from build123d import *

# Parameters (mm, degrees)
F1_DEPTH = 3.175


# Not quite as in the source:
# - a feature names something its author has since deleted; it is built from what else it names


with BuildPart() as f1:
    # F0 (on Front) → F1 (new body)
    with BuildSketch(Plane.XZ):
        with BuildLine():
            ThreePointArc((0, 3.05), (2.1566756826, 2.1566756826), (3.05, 0))
            ThreePointArc((3.05, 0), (2.1566756826, -2.1566756826), (0, -3.05))
            Line((0, -3.05), (0, -4.9800602682))
            ThreePointArc((0, -4.9800602682), (5.7417944409, -6.7685559702), (9.4194688927, -11.5268782485))
            ThreePointArc((9.4194688927, -11.5268782485), (10.31824899, -10.0042357535), (10.6308735731, -8.2639737901))
            Line((10.6308735731, -8.2639737901), (10.6308735731, 8.2639737901))
            ThreePointArc((10.6308735731, 8.2639737901), (10.3103808484, 10.0252834336), (9.389988909, 11.5607983065))
            ThreePointArc((9.389988909, 11.5607983065), (5.7274768906, 6.8026828494), (0, 5))
            Line((0, 5), (0, 3.05))
        make_face()
        with BuildLine():
            ThreePointArc((0, -3.05), (-3.05, 0), (0, 3.05))
            Line((0, 3.05), (0, 5))
            ThreePointArc((0, 5), (-5.7423447428, 6.8130911295), (-9.4024106226, 11.5949046291))
            ThreePointArc((-9.4024106226, 11.5949046291), (-10.3983579477, 10.0170839844), (-10.7465008538, 8.183992176))
            Line((-10.7465008538, 8.183992176), (-10.7465008538, -8.183992176))
            ThreePointArc((-10.7465008538, -8.183992176), (-10.3930329558, -10.0305401514), (-9.3826050837, -11.6160099542))
            ThreePointArc((-9.3826050837, -11.6160099542), (-5.739751248, -6.8156278258), (0, -4.9800602682))
            Line((0, -4.9800602682), (0, -3.05))
        make_face()
        with BuildLine():
            ThreePointArc((-9.4024106226, 11.5949046291), (-5.7423447428, 6.8130911295), (0, 5))
            Line((0, 5), (0, 15))
            ThreePointArc((0, 15), (-4.5199654888, 14.3027938523), (-8.6197512808, 12.275988264))
            ThreePointArc((-8.6197512808, 12.275988264), (-9.0287945556, 11.9558018286), (-9.4024106226, 11.5949046291))
        make_face()
        with BuildLine():
            Line((0, 15), (0, 5))
            ThreePointArc((0, 5), (5.7274768906, 6.8026828494), (9.389988909, 11.5607983065))
            ThreePointArc((9.389988909, 11.5607983065), (8.9445660683, 12.0082283284), (8.4463103597, 12.3959606852))
            ThreePointArc((8.4463103597, 12.3959606852), (4.4193093195, 14.3342144933), (0, 15))
        make_face()
        with BuildLine():
            ThreePointArc((9.4194688927, -11.5268782485), (5.7417944409, -6.7685559702), (0, -4.9800602682))
            Line((0, -4.9800602682), (0, -15))
            ThreePointArc((0, -15), (4.4193093195, -14.3342144933), (8.4463103597, -12.3959606852))
            ThreePointArc((8.4463103597, -12.3959606852), (8.9613594363, -11.9932986506), (9.4194688927, -11.5268782485))
        make_face()
        with BuildLine():
            Line((0, -15), (0, -4.9800602682))
            ThreePointArc((0, -4.9800602682), (-5.739751248, -6.8156278258), (-9.3826050837, -11.6160099542))
            ThreePointArc((-9.3826050837, -11.6160099542), (-9.0178640795, -11.9652859553), (-8.6197512808, -12.275988264))
            ThreePointArc((-8.6197512808, -12.275988264), (-4.5199654888, -14.3027938523), (0, -15))
        make_face()
        with BuildLine():
            ThreePointArc((-8.6197512808, 12.275988264), (-4.5199654888, 14.3027938523), (0, 15))
            ThreePointArc((0, 15), (4.4193093195, 14.3342144933), (8.4463103597, 12.3959606852))
            ThreePointArc((8.4463103597, 12.3959606852), (8.9445660683, 12.0082283284), (9.389988909, 11.5607983065))
            ThreePointArc((9.389988909, 11.5607983065), (9.8463162932, 13.2535592037), (10, 15))
            ThreePointArc((10, 15), (-1.7285678717, 24.8494696869), (-9.4024106226, 11.5949046291))
            ThreePointArc((-9.4024106226, 11.5949046291), (-9.0287945556, 11.9558018286), (-8.6197512808, 12.275988264))
        make_face()
        with BuildLine():
            ThreePointArc((8.4463103597, -12.3959606852), (4.4193093195, -14.3342144933), (0, -15))
            ThreePointArc((0, -15), (-4.5199654888, -14.3027938523), (-8.6197512808, -12.275988264))
            ThreePointArc((-8.6197512808, -12.275988264), (-9.0178640795, -11.9652859553), (-9.3826050837, -11.6160099542))
            ThreePointArc((-9.3826050837, -11.6160099542), (-1.6724608086, -24.8332220833), (10.0345902517, -14.9800004438))
            ThreePointArc((10.0345902517, -14.9800004438), (9.8796089518, -13.2262596432), (9.4194688927, -11.5268782485))
            ThreePointArc((9.4194688927, -11.5268782485), (8.9613594363, -11.9932986506), (8.4463103597, -12.3959606852))
        make_face()
    extrude(amount=F1_DEPTH)


solid = f1.part
Model file for the job. Use its own axes, mm. A direction names the side the tool comes from. Give positions to 0.01 mm unless a question says otherwise; leave off trailing zeros. Loops run counter-clockwise (first coordinate to the right, second up) from the corner with the lowest first, then second, coordinate; pieces in that order, holes last. Notation, with made-up numbers: (59.5, 72) -> (90.5, 72) arc R17 cw to (90.5, 83) -> close; hole circle Ø7 at (22.5, 66). An arc over 180 degrees is marked (long way). Use a Markdown table: item, result. Add a question column.
(1) Slice it at B-B on z = -16.5. List the corners of the cut face in (x, y) (3 decimals), and give its area (3 significant figures).
(2) Slice it at A-A on y = -2. List the corners of the cut face in (x, z).
(3) Slice it at C-C on x = -3.5. List the corners of the cut face in (y, z) (1 decimal).
(4) Tool access for faces 3 (the flat face through (10.631, -2, 0)), 4 (the cylindrical face through (10.31, -1.57, -10.03)), 5 (the cylindrical face through (-10.39, -1.57, 10.04)): list every direction of +Z, -Z, +X, -X, +Y, -Y with a clear straight run to the whole face (end or side of a thin tool).
(5) Mould opens along Z. For faces 1 (the cylindrical face through (-10.4, -1.57, -10.01)), 2 (the flat face through (5, -3.175, 0)) say: +Z half, -Z half, draft (parallel to the pull), parting line (faces both ways), or undercut.
(6) Wall check: line 1 along X through (y, z) = (-0.7, 1); line 2 along Z through (x, y) = (0.5, -0.2); line 3 along Z through (x, y) = (-0.75, -1.05). Give the ranges that are in metal, low to high.
(7) Drop a flat-ended pin along its axis: pin 1 Ø1 at (x, y) = (1.5, -2) entering from +Z. Give the stop position or say it passes through.
Filled sheet:
| question | item | result |
|---|---|---|
| 1 | outline | (-9.849, -3.175) -> (9.918, -3.175) -> (9.918, 0) -> (-9.849, 0) -> close |
| 1 | area | 62.8 mm2 |
| 2 | outline | (-10.75, -8.18) arc R5 ccw to (-9.38, -11.62) arc R10 ccw (long way) to (9.42, -11.53) arc R5 ccw to (10.63, -8.26) -> (10.63, 8.26) arc R5 ccw to (9.39, 11.56) arc R10 ccw (long way) to (-9.4, 11.59) arc R5 ccw to (-10.75, 8.18) -> close; hole circle Ø6.1 at (0, 0) |
| 3 | outline | (-3.2, -24.3) -> (0, -24.3) -> (0, 24.4) -> (-3.2, 24.4) -> close |
| 4 | face 3 | +Z, -Z, +X, +Y, -Y |
| 4 | face 4 | +X, +Y, -Y |
| 4 | face 5 | -X, +Y, -Y |
| 5 | face 1 | undercut |
| 5 | face 2 | draft |
| 6 | line 1 | -10.75 to -2.88, 2.88 to 10.63 |
| 6 | line 2 | -24.97 to -3.01, 3.01 to 24.99 |
| 6 | line 3 | -24.95 to -2.96, 2.96 to 24.97 |
| 7 | pin 1 | z = 24.95 |
